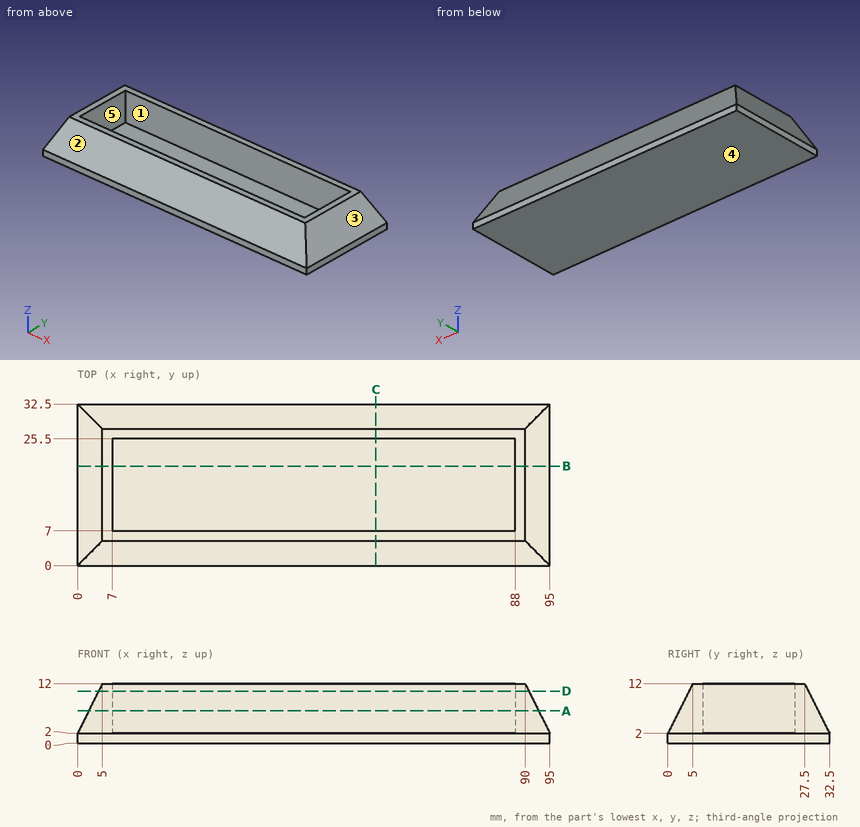
The drawing under review shows one solid part. Ordinate dimensions are in mm from its lowest x, y, z. A direction names the side the tool comes from. Coordinates: 2 decimals unless noted, no trailing zeros. Write each loop counter-clockwise with the first axis right and the second up, starting at its lowest first coordinate (ties: lowest second). Pieces come first, ordered by that corner, then holes. Notation, with made-up numbers: M 68.25,44.5 L 125.25,44.5 A24 cw 125.25,69.5 Z; hole C 33,23.5 d7. An arc over 180 degrees is marked long. Put each result on its own line as item: value.
1) Add section A-A on z = 6.5. Give the boundary of the cut face in (x, y), then the cut area to 3 significant figures.
Computed:
outline: M 2.25,2.25 L 92.75,2.25 L 92.75,30.25 L 2.25,30.25 Z; hole M 7,7 L 88,7 L 88,25.5 L 7,25.5 Z
area: 1,040 mm2
2) Add section D-D on z = 10.5. Give the boundary of the cut face in (x, y), then the cut area to 4 significant figures.
Computed:
outline: M 4.25,4.25 L 90.75,4.25 L 90.75,28.25 L 4.25,28.25 Z; hole M 7,7 L 88,7 L 88,25.5 L 7,25.5 Z
area: 577.5 mm2
3) Add section C-C on x = 60. Give the boundary of the cut face in (y, z).
Computed:
outline: M 0,0 L 32.5,0 L 32.5,2 L 27.5,12 L 25.5,12 L 25.5,2 L 7,2 L 7,12 L 5,12 L 0,2 Z
4) Clearance check with flat-ended pins moving along their axes: pin 1 Ø1 at (y, z) = (6, 5) entering from -X; pin 2 Ø6 at (y, z) = (6, 5.5) entering from +X; pin 3 Ø5.5 at (x, y) = (66, 14.5) entering from +Z. State where each tip first meets the part, or that it passes through.
Computed:
pin 1: stops at x = 1.25
pin 2: stops at x = 94.75
pin 3: stops at z = 2
5) For the marked faces 4 and 5, list the 3-axis set-ups (+Z, -Z, +X, -X, +Y, -Y) from which the entire face can be reached by the end or side of a thin tool; tool diameter is ignored.
Computed:
face 4: -Z, +X, -X, +Y, -Y
face 5: +Z
6) Draft analysis for pull direction X (two halves, no side actions). For the marked faces 1, 2 and 3, state which applies: released by +X, released by -X, zero draft, split by the parting line, or undercut.
Computed:
face 1: undercut
face 2: zero draft
face 3: released by +X
7) Add section B-B on y = 20. Give the boundary of the cut face in (x, z).
Computed:
outline: M 0,0 L 95,0 L 95,2 L 90,12 L 88,12 L 88,2 L 7,2 L 7,12 L 5,12 L 0,2 Z
8) Wall thickness on probe 1 along X at (y, z) = (18, 7); probe 2 along Z at (x, y) = (82.5, 25); probe 3 along X at (y, z) = (22, 9.25) (3 decimals): over which ranges is each line inside the solid? List them lowest first. Write a range as [from, to].
Computed:
probe 1: x = [2.5, 7], [88, 92.5]
probe 2: z = [0, 2]
probe 3: x = [3.625, 7], [88, 91.375]
